Autodesk Fusion 360 part; units mm, degrees
sketch "Sketch1" plane through (0, 0, 0) normal (0, 0, 1) x (1, 0, 0) in component "Display"
  line L0 (0, 0) -> (164, 0)
  line L1 (164, 0) -> (164, 100)
  line L2 (164, 100) -> (0, 100)
  line L3 (0, 100) -> (0, 0)
  dimension "d1" = 164
  dimension "d2" = 100
extrude "Extrude1" add sketch "Sketch1" along normal blind 4 in component "Display"
fillet "Fillet1" radius 1 12 edges at (164, 100, 2) (164, 50, 0) (82, 100, 4) (0, 0, 2) (164, 50, 4) (0, 50, 4) (82, 0, 4) (82, 0, 0) (0, 50, 0) (164, 0, 2) (82, 100, 0) (0, 100, 2) in component "Display"
sketch "Sketch2" plane through (0, 0, 4) normal (0, 0, 1) x (-1, 0, 0) in component "Display"
  line L0 (-163, -99) -> (-1, -99)
  line L1 (-1, -99) -> (-1, -1)
  line L2 (-1, -1) -> (-163, -1)
  line L3 (-163, -1) -> (-163, -99)
  line L4 (-1.81, -96.43) -> (-158.51, -96.43)
  line L5 (-158.51, -96.43) -> (-158.51, -7.33)
  line L6 (-158.51, -7.33) -> (-1.81, -7.33)
  line L7 (-1.81, -7.33) -> (-1.81, -96.43)
  line L8 (-164, -100) -> (0, -100)
  line L9 (-164, 0) -> (-164, -100)
  line L10 (-75.16, -7.33) -> (-85.16, -7.33)
  line L11 (-85.16, -7.33) -> (-85.16, -3.33)
  line L12 (-85.16, -3.33) -> (-75.16, -3.33)
  line L13 (-75.16, -3.33) -> (-75.16, -7.33)
  line L14 (-80.16, -3.33) -> (-80.16, -7.33) construction
  dimension "d7" = 3.57
  dimension "d8" = 5.49
  dimension "d9" = 156.7
  dimension "d10" = 89.1
  dimension "d13" = 10
  dimension "d14" = 4
extrude "Extrude2" cut sketch "Sketch2" against normal blind 0.2 contours L4 L5 L6 L7 L10 | L6 L10 L11 L12 L13 in component "Display"
component "Display" placed x (1, 0, 0) y (0, 1, 0) z (0, 0, 1) at (0, 0, 0)
Part model, mm, in its own coordinate system. Round coordinates to 2 decimals unless told otherwise and drop trailing zeros. Loops run counter-clockwise (first coordinate to the right, second up) from the corner with the lowest first, then second, coordinate; pieces in that order, holes last. Notation, with made-up numbers: (75, 47) -> (106, 47) arc R25 cw to (106, 60) -> close; hole circle Ø10 at (53.25, 25.25). An arc over 180 degrees is marked (long way). Use one line per item in the form item = value. Start each with the question number.
Item 1: Band-saw the part on B-B (y = 31). List the corners of the cut face in (x, z), plus the area to 3 significant figures.
Item 2: Two-plate mould, pull along X, no slides. Class faces 1 (the flat face through (94, 7, 4)), 2 (the flat face through (81, 49, 3.8)): released by +X, released by -X, zero draft, split by the parting line, or undercut.
Item 3: Drill centre lines: line 1 along Z through (x, y) = (49, 95); line 2 along Y through (x, z) = (27.5, 0.9); line 3 along X through (y, z) = (43.5, 3.05). Where is each one in solid material? Low to high.
Item 4: Band-saw the part on A-A (x = 152.5). List the corners of the cut face in (y, z), plus the area to 3 significant figures.
Item 5: Drop a flat-ended pin along its axis: pin 1 Ø12 at (x, y) = (43.5, 59.5) entering from +Z. Give the stop position or say it passes through.
Data:
q1.outline = (0, 1) arc R1 ccw to (1, 0) -> (163, 0) arc R1 ccw to (164, 1) -> (164, 3) arc R1 ccw to (163, 4) -> (158.51, 4) -> (158.51, 3.8) -> (1.81, 3.8) -> (1.81, 4) -> (1, 4) arc R1 ccw to (0, 3) -> close
q1.area = 624 mm^2
q2.face_1 = zero draft
q2.face_2 = undercut
q3.line_1 = 0 to 3.8
q3.line_2 = 0.01 to 99.99
q3.line_3 = 0 to 164
q4.outline = (0, 1) arc R1 ccw to (1, 0) -> (99, 0) arc R1 ccw to (100, 1) -> (100, 3) arc R1 ccw to (99, 4) -> (96.43, 4) -> (96.43, 3.8) -> (7.33, 3.8) -> (7.33, 4) -> (1, 4) arc R1 ccw to (0, 3) -> close
q4.area = 381 mm^2
q5.pin_1 = 3.8
